Could you check a few things on this model? Use its own coordinates, in mm. Round coordinates to 2 decimals unless told otherwise and drop trailing zeros. Loops run counter-clockwise (first coordinate to the right, second up) from the corner with the lowest first, then second, coordinate; pieces in that order, holes last. Notation, with made-up numbers: M 1,-40 L 55,-40 A14 ccw 55,-17 Z; hole C 62,84 d6. An arc over 180 degrees is marked long. Answer in a Markdown table with one row per item.
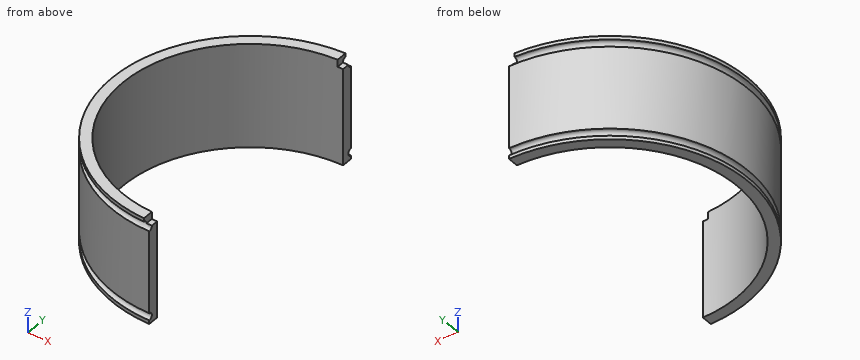
```python
from build123d import *

# Parameters (mm, degrees)
MAIN_SHELL_DEPTH = 29
END_STOP_DEPTH   = 2


with BuildPart() as part:
    # Sketch1 → Main Shell (new body)
    with BuildSketch(Plane.XY):
        with BuildLine():
            Line((0, 38.5), (0, 35.5))
            ThreePointArc((0, 35.5), (-35.5, 0), (0, -35.5))
            Line((0, -35.5), (0, -38.5))
            ThreePointArc((0, -38.5), (-38.5, 0), (0, 38.5))
        make_face()
    extrude(amount=MAIN_SHELL_DEPTH)

    # Sketch3 → Rubber Band Holder (revolve, cut)
    with BuildSketch(Plane(origin=(0, 0, 0), x_dir=(0, 0, -1), z_dir=(1, 0, 0))):
        with BuildLine():
            Line((-28, 38.5), (-26, 38.5))
            ThreePointArc((-26, 38.5), (-27, 37.5), (-28, 38.5))
        make_face()
        with BuildLine():
            Line((-3, 38.5), (-1, 38.5))
            ThreePointArc((-1, 38.5), (-2, 37.5), (-3, 38.5))
        make_face()
    revolve(axis=Axis((0, 0, 29), (0, 0, -1)), mode=Mode.SUBTRACT)

    # Sketch4 → End Stop (cut)
    with BuildSketch(Plane.XY.offset(29)):
        with BuildLine():
            Line((0, 38.5), (0, 35.5))
            ThreePointArc((0, 35.5), (-0.750167508, 35.49207304), (-1.5, 35.468295702))
            Line((-1.5, 35.468295702), (-1.5, 38.470768123))
            ThreePointArc((-1.5, 38.470768123), (-0.750142404, 38.492691337), (0, 38.5))
        make_face()
        with BuildLine():
            Line((-1.5, -38.470768123), (-1.5, -35.468295702))
            ThreePointArc((-1.5, -35.468295702), (-0.750167508, -35.49207304), (0, -35.5))
            Line((0, -35.5), (0, -38.5))
            ThreePointArc((0, -38.5), (-0.750142404, -38.492691337), (-1.5, -38.470768123))
        make_face()
    extrude(amount=-END_STOP_DEPTH, mode=Mode.SUBTRACT)


solid = part.part
```
1) Will these pins go through, and if not, where does the flat tip stop? P1, Ø1.5, axis at y = -22.5, z = 9, coming from the +X side; P2, Ø4, axis at x = -30.5, y = 11, coming from the +Z side; P3, Ø1.5, axis at y = -15, z = 7, coming from the -X side; P4, Ø5, axis at y = 18, z = 16, coming from the -X side.
Computed:
| item | result |
|---|---|
| P1 | stops at x = -26.83 |
| P2 | passes through |
| P3 | stops at x = -35.77 |
| P4 | stops at x = -35.24 |
2) I want a section at B-B, the plane z = 23.5. Please give me the cut outline in (x, y), plus the area to 3 significant figures.
Computed:
| item | result |
|---|---|
| outline | M 0,-38.5 L 0,-35.5 A35.5 cw 0,35.5 L 0,38.5 A38.5 ccw Z |
| area | 349 mm² |
3) I want a section at A-A, the plane y = 0. Please give me the cut outline in (x, z).
Computed:
| item | result |
|---|---|
| outline | M -38.5,0 L -35.5,0 L -35.5,29 L -38.5,29 L -38.5,28 A1 cw -38.5,26 L -38.5,3 A1 cw -38.5,1 Z |
4) I need wall thicknesses on line 1 (Y direction, x = -18.5, z = 11); line 2 (Z direction, x = -24, y = -29); line 3 (Y direction, x = -31, z = 18.25). Which ranges of each line are inside material? Lowest first, please.
Computed:
| item | result |
|---|---|
| line 1 | y = -33.76 to -30.3, 30.3 to 33.76 |
| line 2 | z = 0 to 1.48, 2.52 to 26.48, 27.52 to 29 |
| line 3 | y = -22.83 to -17.3, 17.3 to 22.83 |
